Check sheet for the modelled part. Datum: model origin and axes. Units: mm. Round coordinates to 2 decimals unless told otherwise and drop trailing zeros. Write each loop counter-clockwise with the first axis right and the second up, starting at its lowest first coordinate (ties: lowest second). Pieces come first, ordered by that corner, then holes. Notation, with made-up numbers: (-12.75, 83.5) -> (45.25, 83.5) arc R22 ccw to (45.25, 112.5) -> close; hole circle Ø6 at (43.25, 6.25). An arc over 180 degrees is marked (long way). One line per item, written item: value.
Autodesk Inventor part; units mm, degrees
ref_plane "YZ Plane" through (0, 0, 0) normal (1, 0, 0) x (0, 1, 0)
ref_plane "XZ Plane" through (0, 0, 0) normal (0, 1, 0) x (-1, 0, 0)
ref_plane "XY Plane" through (0, 0, 0) normal (0, 0, 1) x (1, 0, 0)
sketch "Sketch1" plane through (0, 0, 0) normal (0, 0, 1) x (1, 0, 0)
  line L0 (-28.575, 19.05) -> (28.575, 19.05)
  line L1 (28.575, 19.05) -> (28.575, -19.05)
  line L2 (28.575, -19.05) -> (-28.575, -19.05)
  line L3 (-28.575, -19.05) -> (-28.575, 19.05)
  circle A0 centre (0, 0) radius 9.525
  circle A1 centre (0, 0) radius 15.875
  line L4 (-26.3525, 9.525) -> (-21.2725, 9.525)
  line L5 (-21.2725, 9.525) -> (-21.2725, -9.525)
  line L6 (-21.2725, -9.525) -> (-26.3525, -9.525)
  line L7 (-26.3525, -9.525) -> (-26.3525, 9.525)
  arc A2 (-21.2725, 9.525) -> (-26.3525, 9.525) centre (-23.8125, 9.525) ccw
  arc A3 (-26.3525, -9.525) -> (-21.2725, -9.525) centre (-23.8125, -9.525) ccw
  line L8 (21.2725, 9.525) -> (26.3525, 9.525)
  line L9 (26.3525, 9.525) -> (26.3525, -9.525)
  line L10 (26.3525, -9.525) -> (21.2725, -9.525)
  line L11 (21.2725, -9.525) -> (21.2725, 9.525)
  arc A4 (26.3525, 9.525) -> (21.2725, 9.525) centre (23.8125, 9.525) ccw
  arc A5 (21.2725, -9.525) -> (26.3525, -9.525) centre (23.8125, -9.525) ccw
  point P0 (7.6157, 13.929)
  point P1 (-15.8707, -0.3691)
  point P2 (8.255, -13.5599)
  dimension "d5" = 31.75
  dimension "d0" = 19.05
  dimension "d1" = 19.05
  dimension "d2" = 38.1
  dimension "d3" = 28.575
  dimension "d4" = 57.15
  dimension "d8" = 360
  dimension "d11" = 4.7625
  dimension "d12" = 19.05
  dimension "d13" = 9.525
  dimension "d14" = 5.08
  dimension "d15" = 19.05
  dimension "d16" = 5.08
  dimension "d17" = 4.7625
  dimension "d33" = 8.255
extrude "Extrusion1" add sketch "Sketch1" against normal blind 3.175 contours L0 L1 L2 L3 | A1
hole "Hole1" at (7.6157, 13.929, 0) at (-15.8707, -0.3691, 0) at (8.255, -13.5599, 0) direction (0, 0, -1) diameter 3.2512 end through all
fillet "Fillet1" radius 6.35 4 edges at (28.575, 19.05, -1.5875) (-28.575, 19.05, -1.5875) (-28.575, -19.05, -1.5875) (28.575, -19.05, -1.5875)
equation "\"d4\" = 2 * d3"
equation "\"d17\" = d11"
properties part number "dewalt tom mounting plate"
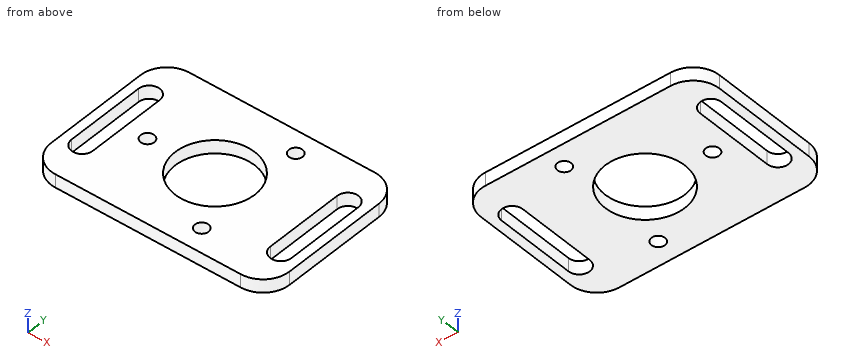
Item 1: Sectioned sample at A-A on x = 0. Enter the section's corners in (y, z) (3 decimals).
Answer:
outline: (-19.05, -3.175) -> (-9.525, -3.175) -> (-9.525, 0) -> (-19.05, 0) -> close; (9.525, -3.175) -> (19.05, -3.175) -> (19.05, 0) -> (9.525, 0) -> close
Item 2: Thickness scan on line 1 (X direction, y = -0.5, z = -1.2) (1 decimal); line 2 (X direction, y = -8.5, z = -2.1) (1 decimal); line 3 (X direction, y = 7, z = -1.15) (1 decimal). Record the ranges inside material, lowest first.
Answer:
line 1: x = -28.6 to -26.4, -21.3 to -17.5, -14.3 to -9.5, 9.5 to 21.3, 26.4 to 28.6
line 2: x = -28.6 to -26.4, -21.3 to -4.3, 4.3 to 21.3, 26.4 to 28.6
line 3: x = -28.6 to -26.4, -21.3 to -6.5, 6.5 to 21.3, 26.4 to 28.6
Item 3: Sectioned sample at B-B on y = 5. Enter the section's corners in (x, z) (1 decimal).
Answer:
outline: (-28.6, -3.2) -> (-26.4, -3.2) -> (-26.4, 0) -> (-28.6, 0) -> close; (-21.3, -3.2) -> (-8.1, -3.2) -> (-8.1, 0) -> (-21.3, 0) -> close; (8.1, -3.2) -> (21.3, -3.2) -> (21.3, 0) -> (8.1, 0) -> close; (26.4, -3.2) -> (28.6, -3.2) -> (28.6, 0) -> (26.4, 0) -> close
Item 4: Depth check by flat-ended pin: P1, Ø1.5, axis at x = -12.5, y = -10, coming from the +Z side. Enter the tip coordinate at first touch or a pass-through.
Answer:
P1: stops at z = 0
Item 5: Sectioned sample at C-C on y = 15. Enter the section's corners in (x, z) (3 decimals), and give its area (3 significant figures).
Answer:
outline: (-28.144, -3.175) -> (6.393, -3.175) -> (6.393, 0) -> (-28.144, 0) -> close; (8.839, -3.175) -> (28.144, -3.175) -> (28.144, 0) -> (8.839, 0) -> close
area: 171 mm^2
Item 6: Sectioned sample at D-D on z = -1.35. Count the separate pieces of the cut face and the enclosed holes in it, and give its area (3 significant figures).
Answer:
separate pieces: 1
enclosed holes: 6
area: 1,600 mm^2
